Autodesk Fusion 360 part; units mm, degrees
sketch "Sketch1" plane through (0, 0, 0) normal (1, 0, 0) x (0, 1, 0)
  line L0 (10, -10.35) -> (-10, -10.35)
  line L1 (-10, -10.35) -> (-10, 10.35)
  line L2 (-10, 10.35) -> (10, 10.35)
  line L3 (10, 10.35) -> (10, -10.35)
  line L4 (10, -10.35) -> (-10, 10.35) construction
  line L5 (-10, -10.35) -> (10, 10.35) construction
  line L6 (12.9717, -13.35) -> (-12.9717, -13.35)
  line L7 (-12.9717, -13.35) -> (-12.9717, 13.35)
  line L8 (-12.9717, 13.35) -> (12.9717, 13.35)
  line L9 (12.9717, 13.35) -> (12.9717, -13.35)
  line L10 (12.9717, -13.35) -> (-12.9717, 13.35) construction
  line L11 (-12.9717, -13.35) -> (12.9717, 13.35) construction
  line L12 (10, 10.35) -> (12.9717, 10.35)
  line L13 (-10, 10.35) -> (-12.9717, 10.35)
  line L14 (-10, -10.35) -> (-12.9717, -10.35)
  line L15 (-12.9717, -10.35) -> (12.9717, -10.35)
  dimension "d1" = 20
  dimension "d2" = 20.7
  dimension "d3" = 26.7
extrude "Extrude1" add sketch "Sketch1" along normal blind 20 contours L0 L6 L7 L9 L14 L15 | L2 L7 L8 L9 L12 L13 makes body 1 at (6.6667, -4.3239, 10.35) makes body 2 at (13.3333, -4.3239, -10.35)
extrude "Extrude2" add sketch "Sketch1" against normal blind 4 separate body contours L0 L1 L2 L3 L15 | L3 L9 L12 L15 | L1 L7 L13 L14 L15 makes body 3
extrude "Extrude3" add sketch "Sketch1" against normal blind 4 contours L0 L6 L7 L9 L14 L15 | L2 L7 L8 L9 L12 L13 bodies 1 2 3
sketch "Sketch2" plane through (0, 0, 13.35) normal (0, 0, 1) x (-1, 0, 0)
  line L0 (4, 12.9717) -> (-20, 12.9717)
  line L1 (-20, 12.9717) -> (-20, -12.9717)
  line L2 (-20, -12.9717) -> (4, -12.9717)
  line L3 (4, -12.9717) -> (4, 12.9717)
  line L4 (4, 0) -> (26, 0)
  circle A0 centre (26, 0) radius 19.55
  circle A1 centre (26, 0) radius 14 construction
  circle A2 centre (26, 0) radius 15.25 construction
  line L5 (26, 0) -> (26, -14)
  circle A3 centre (26, 0) radius 21.5
  line L6 (4, -12.9717) -> (16.3028, -19.1889)
  line L7 (4, 12.9717) -> (16.3028, 19.1889)
  circle A4 centre (26, 0) radius 10.05
  line L8 (-20, -12.9717) -> (-9.5, -12.9717)
  line L9 (-9.5, -12.9717) -> (-9.5, -8.8717)
  circle A5 centre (-9.5, -8.8717) radius 1.6
  line L10 (4, 0) -> (-20, 0) construction
  circle A6 centre (-9.5, 8.8717) radius 1.6
  line L11 (16.3028, -19.1889) -> (16.3028, 19.1889)
  line L12 (26, 0) -> (37.486, -8.0426)
  circle A7 centre (37.486, -8.0426) radius 1.56
  circle A8 centre (27.2221, 13.9685) radius 1.56
  circle A9 centre (13.2919, -5.9259) radius 1.56
  line L13 (26, 0) -> (25.9989, 0)
  line L14 (26, 0) -> (41.25, 0.3993)
  line L15 (26, 0) -> (41, 0) construction
  circle A10 centre (41.25, 0.3993) radius 1.56
  circle A11 centre (18.0292, 13.0072) radius 1.56
  circle A12 centre (18.7208, -13.4066) radius 1.56
  dimension "d22" = 22
  dimension "d23" = 39.1
  dimension "d24" = 28
  dimension "d25" = 30.5
  dimension "d26" = 14
  dimension "d32" = 43
  dimension "d33" = 20.1
  dimension "d38" = 10.5
  dimension "d39" = 4.1
  dimension "d40" = 3.2
  dimension "d56" = 3.12
  dimension "d66" = 1.5
  dimension "d67" = 3.12
  dimension "d68" = 15.25
  dimension "d70" = 360
extrude "Extrude4" add sketch "Sketch2" against normal blind 2 separate body contours L4 A0 A4 L11 | A0 A4 L11 | L4 A0 A4 L11 makes body 4
extrude "Extrude5" add sketch "Sketch2" against normal blind 30 contours L3 L4 A3 L7 | L3 L4 A3 L6 | L4 A0 A3 L11 | L4 A0 A3 L11 bodies 1 4
extrude "Extrude6" cut sketch "Sketch2" against normal blind 34 contours A5 | A6 bodies 1
extrude "Extrude7" add sketch "Sketch2" against normal blind 20 contours A0 A3 L11 bodies 1
equation "d68 = ( 30.5 / 2 ) * 1 mm"
CAD build for the part. Positions are in the model's coordinates, mm. A direction names the side the tool comes from. Coordinates: 2 decimals unless noted, no trailing zeros. Order: outer loops, then holes, each group sorted by start corner. A loop starts at its lowest first (then second) coordinate and runs counter-clockwise, first axis right, second up. Notation, with made-up numbers: (34.25, 8.25) -> (48.25, 8.25) arc R30 ccw to (48.25, 31.25) -> close; hole circle Ø11 at (29.25, 89). An arc over 180 degrees is marked (long way). Use one line per item in the form item = value. Start each with the question number.
1) Band-saw the part on A-A on x = 5. Give the cut face in (y, z).
2) Drill centre lines: L1, parallel to Y at x = 9.5, z = -12.55; L2, parallel to Z at x = 16.5, y = 5.5; L3, parallel to Z at x = -13, y = 8. Where is each one in solid material? Low to high. Write a range as [from, to].
3) Band-saw the part on B-B on z = -4.75. Give the cut face in (x, y).
4) Tool access for faces 4 (the flat face through (-0.2, 12.972, 0.2)), 5 (the flat face through (8, 0, -13.35)), 6 (the flat face through (-16.303, -18, -12)): list every direction of +Z, -Z, +X, -X, +Y, -Y with a clear straight run to the whole face (end or side of a thin tool).
5) Band-saw the part on C-C on y = -3. Give the cut face in (x, z).
6) Band-saw the part on D-D on x = -28. Give the cut face in (y, z), then the cut area to 3 significant figures.
7) Drop flat-ended pins along their axis: pin 1 (1.9 mm diameter, centred on x = -27.22, y = -13.97, fed in from -Z); pin 2 (1.5 mm diameter, centred on x = -14.5, z = -1.5, fed in from -Y); pin 3 (4 mm diameter, centred on x = -13.29, y = 5.93, fed in from -Z); pin 4 (1.5 mm diameter, centred on y = -16.5, z = -6, fed in from -X). Give the stop position or say it passes through.
8) Pull direction Y, two halves, no side cores. Call faces 1 (the cylindrical face through (-6.47, -0.86, 0.66)), 2 (the flat face through (-16.303, 18, -12)), 3 (the flat face through (-10.07, -16.04, -1.44)): +Y half, -Y half, draft (parallel to the pull), parting line (faces both ways), or undercut.
Entries:
q1.outline = (-12.97, -13.35) -> (12.97, -13.35) -> (12.97, -10.35) -> (-12.97, -10.35) -> close; (-12.97, 10.35) -> (12.97, 10.35) -> (12.97, 13.35) -> (-12.97, 13.35) -> close
q2.L1 = [-12.97, -10.47], [-7.27, 7.27], [10.47, 12.97]
q2.L2 = [-13.35, -10.35], [10.35, 13.35]
q2.L3 = [11.35, 13.35]
q3.outline = (-16.3, -19.19) -> (-4, -12.97) -> (0, -12.97) -> (0, 12.97) -> (-4, 12.97) -> (-16.3, 19.19) arc R21.5 ccw (long way) to start; hole circle Ø39.1 at (-26, 0)
q4.face_4 = +Z, -Z, +X, +Y
q4.face_5 = -Z, +X, +Y, -Y
q4.face_6 = -Z, -X, +Y, -Y
q5.outline = (-47.29, -6.65) -> (-45.32, -6.65) -> (-45.32, 11.35) -> (-35.59, 11.35) -> (-35.59, 13.35) -> (-47.29, 13.35) -> close; (-16.41, 11.35) -> (-6.68, 11.35) -> (-6.68, -16.65) -> (-4, -16.65) -> (-4, -13.35) -> (20, -13.35) -> (20, -10.35) -> (0, -10.35) -> (0, 10.35) -> (20, 10.35) -> (20, 13.35) -> (-16.41, 13.35) -> close
q6.outline = (-21.41, -6.65) -> (-19.45, -6.65) -> (-19.45, 11.35) -> (-15.32, 11.35) -> (-15.32, 13.35) -> (-21.41, 13.35) -> close; (-12.62, 11.35) -> (-9.85, 11.35) -> (-9.85, 13.35) -> (-12.62, 13.35) -> close; (9.85, 11.35) -> (19.45, 11.35) -> (19.45, -6.65) -> (21.41, -6.65) -> (21.41, 13.35) -> (9.85, 13.35) -> close
q6.area = 111 mm2
q7.pin_1 = through
q7.pin_2 = -18.66
q7.pin_3 = 11.35
q7.pin_4 = -40.64
q8.face_1 = undercut
q8.face_2 = draft
q8.face_3 = -Y half
